Autodesk Inventor part; units mm, degrees
ref_plane "YZ Plane" through (0, 0, 0) normal (1, 0, 0) x (0, 1, 0)
ref_plane "XZ Plane" through (0, 0, 0) normal (0, 1, 0) x (-1, 0, 0)
ref_plane "XY Plane" through (0, 0, 0) normal (0, 0, 1) x (1, 0, 0)
sketch "Sketch1" plane through (0, 0, 0) normal (0, 0, 1) x (1, 0, 0)
  line L0 (118.7984, -15.7076) -> (118.7984, -63.6601)
  line L1 (118.7984, -63.6601) -> (108.7984, -63.6601)
  line L2 (108.7984, -63.6601) -> (108.7984, -15.7076)
  line L3 (108.7984, -15.7076) -> (118.7984, -15.7076)
  line L4 (114.7984, 76.5) -> (114.7984, -850)
  point P0 (0, 0)
  dimension "d0" = 6
  dimension "d1" = 10
extrude "Extrusion1" add sketch "Sketch1" along normal mid plane 10
fillet "Fillet1" radius 8.35 2 edges at (108.7984, -15.7076, 0) (108.7984, -63.6601, 0)
fillet "Fillet2" radius 2 2 edges at (118.7984, -39.6839, -5) (118.7984, -39.6839, 5)
sketch "Sketch2" plane through (108.7984, -55.3101, 5) normal (-1, 0, 0) x (0, 0, 1)
  line L0 (-10, 31.2524) -> (0, 31.2524)
  line L1 (-6, 25.2524) -> (-4, 25.2524)
  line L2 (-4, 25.2524) -> (-4, 19.2524)
  line L3 (-4, 19.2524) -> (-6, 19.2524)
  line L4 (-6, 19.2524) -> (-6, 25.2524)
  line L5 (-5, 424.5751) -> (-5, -1099.7802)
  line L6 (-6, 15.2524) -> (-4, 15.2524)
  line L7 (-4, 15.2524) -> (-4, 9.2524)
  line L8 (-4, 9.2524) -> (-6, 9.2524)
  line L9 (-6, 9.2524) -> (-6, 15.2524)
  line L10 (-6.5, 55.3101) -> (-3.5, 55.3101)
  line L11 (-3.5, -794.6899) -> (-3.5, 55.3101)
  line L12 (-6.5, -794.6899) -> (-3.5, -794.6899)
  line L13 (-6.5, -794.6899) -> (-6.5, 55.3101)
  point P0 (-5, 55.3101)
  dimension "d6" = 1
  dimension "d7" = 2
  dimension "d8" = 6
  dimension "d9" = 6
  dimension "d12" = 10
extrude "Extrusion2" add sketch "Sketch2" along normal blind 35.4 contours L5 L3 L4 L1 | L1 L2 L3 L5 | L8 L9 L6 L5 | L5 L6 L7 L8
sketch "Sketch3" plane through (0, 0, 5) normal (0, 0, 1) x (1, 0, 0)
  line L0 (108.7984, -55.3101) -> (108.7984, -24.0576)
  circle A0 centre (114.2984, -37.715) radius 3
  point P0 (116.7984, -15.715)
  point P1 (0, 0)
  dimension "d19" = 5.5
  dimension "d20" = 22
  dimension "d23" = 6
extrude "Extrusion3" add sketch "Sketch3" along normal mid plane 5
properties part number "ThreadBreak"
Geometry: final body of the model. Coordinates: model frame, mm. A direction names the side the tool comes from. Give positions to 0.01 mm unless a question says otherwise; leave off trailing zeros. Write each loop counter-clockwise with the first axis right and the second up, starting at its lowest first coordinate (ties: lowest second). Pieces come first, ordered by that corner, then holes. Notation, with made-up numbers: (42.5, 38.5) -> (47.5, 38.5) arc R35 cw to (47.5, 71.5) -> close; hole circle Ø10 at (83.5, -10). An arc over 180 degrees is marked (long way). Answer as a JSON object with one key per item and string values.
1. Mould query, pull axis Y, two halves, no side actions, for faces 4 (the cylindrical face through (111.3, -18.1, 0.1)), 5 (the flat face through (91, -43, -1)), 6 (the flat face through (91, -36.058, 0)). Classes: pulls with the +Y half, pulls with the -Y half, needs draft (parallel to the pull), parting line crosses it, or undercut.
Ans:
{"face 4": "pulls with the +Y half", "face 5": "needs draft", "face 6": "undercut"}
2. Cut plane A-A on x = 96.5. Output: boundary loops of the cut face in (y, z).
Ans:
{"outline": "(-46.06, -1) -> (-40.06, -1) -> (-40.06, 1) -> (-46.06, 1) -> close; (-36.06, -1) -> (-30.06, -1) -> (-30.06, 1) -> (-36.06, 1) -> close"}
3. Cut plane C-C on z = -0.25. Output: boundary loops of the cut face in (x, y).
Ans:
{"outline": "(73.4, -46.06) -> (108.8, -46.06) -> (108.8, -55.31) arc R8.35 ccw to (117.15, -63.66) -> (118.8, -63.66) -> (118.8, -15.71) -> (117.15, -15.71) arc R8.35 ccw to (108.8, -24.06) -> (108.8, -30.06) -> (73.4, -30.06) -> (73.4, -36.06) -> (108.8, -36.06) -> (108.8, -40.06) -> (73.4, -40.06) -> close"}
4. Access query for faces 1 (the flat face through (91, -40.058, 0)), 2 (the flat face through (91, -33, 1)), 3 (the flat face through (91, -33, -1)). Directions: +Z, -Z, +X, -X, +Y, -Y. A direction counts if a zero-diameter tool reaches every point of the face in a straight line with its end or side. Return the directions, or none.
Ans:
{"face 1": "+Z, -Z, -X", "face 2": "+Z, -X, +Y, -Y", "face 3": "-Z, -X, +Y, -Y"}
5. Ray query, probe 1 along Y at (x, z) = (104, 0.75); probe 2 along Z at (x, y) = (113.5, -34.5); probe 3 along Z at (x, y) = (92, -35). Return the intervals inside material, ascending. Write a range as from..to.
Ans:
{"probe 1": "y = -46.06..-40.06, -36.06..-30.06", "probe 2": "z = -5..5", "probe 3": "z = -1..1"}
6. Contact query for flat-ended pins moving along their axis: pin 1 (1 mm diameter, centred on x = 79.5, y = -40.5, fed in from +Z); pin 2 (1.8 mm diameter, centred on x = 92.5, y = -43.5, fed in from -Z); pin 3 (1 mm diameter, centred on x = 94, z = -0.5, fed in from +Y). Output: stop coordinate, or through.
Ans:
{"pin 1": "stops at z = 1", "pin 2": "stops at z = -1", "pin 3": "stops at y = -30.06"}
7. Cut plane B-B on y = -45. Output: boundary loops of the cut face in (x, z), and give its area (3 significant figures).
Ans:
{"outline": "(73.4, -1) -> (108.8, -1) -> (108.8, -5) -> (116.8, -5) arc R2 ccw to (118.8, -3) -> (118.8, 3) arc R2 ccw to (116.8, 5) -> (108.8, 5) -> (108.8, 1) -> (73.4, 1) -> close", "area": "169 mm^2"}
8. Cut plane D-D on x = 115.5. Output: boundary loops of the cut face in (y, z).
Ans:
{"outline": "(-63.5, -5) -> (-15.87, -5) -> (-15.87, 5) -> (-34.97, 5) -> (-34.97, 7.5) -> (-40.46, 7.5) -> (-40.46, 5) -> (-63.5, 5) -> close"}
